```python
from build123d import *

# Parameters (mm, degrees)
F0_W     = 3.683
F0_H     = 3.683
F0_R     = 1.5875
F1_DEPTH = 8.98525
F3_DEPTH = 3.683
F4_R     = 1.84149


# Not quite as in the source:
# - a fillet or chamfer is up to 0.001 mm smaller than in the source, because OpenCascade refuses the exact size


with BuildPart() as f1:
    # F0 (on Top) → F1 (new body)
    with BuildSketch(Plane.XY):
        Rectangle(F0_W, F0_H)
        Circle(F0_R, mode=Mode.SUBTRACT)
    extrude(amount=F1_DEPTH)

    # F2 (on face) → F3 (cut, through all)
    with BuildSketch(Plane.XZ.offset(1.8415)):
        with BuildLine():
            Line((0, 8.98525), (-0.933255592, 8.98525))
            ThreePointArc((-0.933255592, 8.98525), (-0.4836015922, 8.7958842904), (0, 8.73125))
            Line((0, 8.73125), (0, 8.98525))
        make_face()
        with BuildLine():
            Line((0, 8.98525), (0, 8.73125))
            ThreePointArc((0, 8.73125), (0.4836015922, 8.7958842904), (0.933255592, 8.98525))
            Line((0.933255592, 8.98525), (0, 8.98525))
        make_face()
    extrude(amount=-F3_DEPTH, mode=Mode.SUBTRACT)

    # F4 (radius 1.8415 in the source; OpenCascade refuses exactly that, so slightly less here)
    f4_edges = [f1.edges().sort_by_distance(p)[0] for p in [
        (-1.8415, -1.8415, 4.492625),
        (1.8415, -1.8415, 4.492625),
        (1.8415, 1.8415, 4.492625),
        (-1.8415, 1.8415, 4.492625),
    ]]
    fillet(f4_edges, radius=F4_R)


solid = f1.part
```
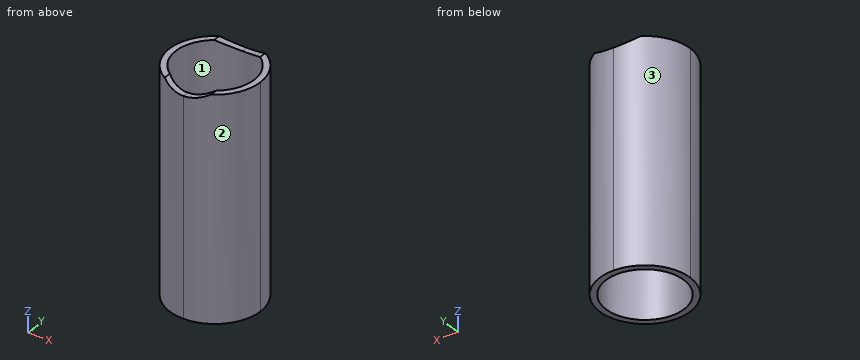
The listing builds one solid part. Answer for the finished solid, in the listing's coordinates (mm). Face numbers are marked on the shaded views. Coordinates: 2 decimals unless noted, no trailing zeros. Write each loop counter-clockwise with the first axis right and the second up, starting at its lowest first coordinate (ties: lowest second). Pieces come first, ordered by that corner, then holes. Notation, with made-up numbers: (-39, -28.5) - (3, -28.5) arc R9 ccw to (3, -19.5) - close; hole circle Ø6 at (-37.75, -36). An arc over 180 degrees is marked (long way). One line per item, written item: value.
1) Find section D-D (y = 1.5). Give the vertices of the cut face in (x, z), and give its area (3 significant figures).
Geometry check:
outline: (-1.07, 0) - (-0.52, 0) - (-0.52, 8.81) arc R1.84 cw to (-0.93, 8.99) - (-1.07, 8.99) - close; (0.52, 0) - (1.07, 0) - (1.07, 8.99) - (0.93, 8.99) arc R1.84 cw to (0.52, 8.81) - close
area: 9.77 mm2
2) Consider line 1 along X through (y, z) = (0, 5.25); line 2 along X through (y, z) = (0.35, 1.75). Determine where each line is inside the solid, lowest interval first. Write a range as from..to.
Geometry check:
line 1: x = -1.84..-1.59, 1.59..1.84
line 2: x = -1.81..-1.55, 1.55..1.81
3) Find section C-C (y = -0.6). Give the vertices of the cut face in (x, z), and give its area (3 significant figures).
Geometry check:
outline: (-1.74, 0) - (-1.47, 0) - (-1.47, 8.99) - (-1.74, 8.99) - close; (1.47, 0) - (1.74, 0) - (1.74, 8.99) - (1.47, 8.99) - close
area: 4.87 mm2
4) Find section B-B (x = -1.1). Give the vertices of the cut face in (y, z).
Geometry check:
outline: (-1.48, 0) - (-1.14, 0) - (-1.14, 8.99) - (-1.48, 8.99) - close; (1.14, 0) - (1.48, 0) - (1.48, 8.99) - (1.14, 8.99) - close
5) For a pull along Y with two mould halves and no side action, classify the marked faces 1, 2 and 3 as pulls with the +Y half, pulls with the -Y half, needs draft (parallel to the pull), parting line crosses it, or undercut.
Geometry check:
face 1: undercut
face 2: pulls with the -Y half
face 3: pulls with the +Y half
